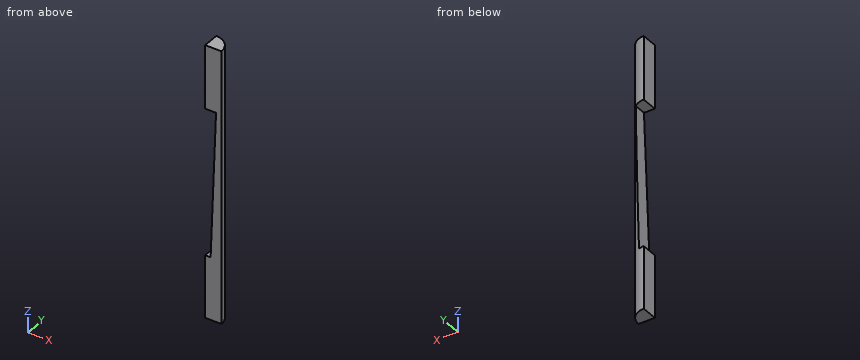
Autodesk Inventor part; units mm, degrees
ref_plane "YZ Plane" through (0, 0, 0) normal (1, 0, 0) x (0, 1, 0)
ref_plane "XZ Plane" through (0, 0, 0) normal (0, 1, 0) x (-1, 0, 0)
ref_plane "XY Plane" through (0, 0, 0) normal (0, 0, 1) x (1, 0, 0)
sketch "Sketch1" plane through (0, 0, 0) normal (0, 0, 1) x (1, 0, 0)
  arc A0 (9.525, 0) -> (0, 9.525) centre (0, 0) ccw
  line L0 (0, 9.525) -> (0, 0)
  line L1 (0, 0) -> (9.525, 0)
  dimension "d0" = 19.05
extrude "Extrusion1" add sketch "Sketch1" along normal mid plane 161.925
sketch "Sketch2" plane through (0, 0, 80.9625) normal (0, -1, 0) x (1, 0, 0)
  line L0 (0, -38.1) -> (6.35, -38.1)
  line L1 (3.175, -123.825) -> (0, -123.825)
  line L2 (0, -123.825) -> (0, -38.1)
  line L3 (9.525, -161.925) -> (0, -161.925)
  line L4 (0, -161.925) -> (0, 0)
  line L5 (3.175, -123.825) -> (6.35, -38.1)
  point P0 (0, -80.9625)
  dimension "d4" = 38.1
  dimension "d8" = 3.175
  dimension "d9" = 6.35
extrude "Extrusion2" cut sketch "Sketch2" against normal through all
sketch "Sketch3" plane through (0, 0, -80.9625) normal (0, -1, 0) x (1, 0, 0)
  line L0 (9.525, 0) -> (0, 0)
  line L1 (0, 0) -> (0, 38.1)
  line L2 (9.525, 0) -> (0, 0)
  line L3 (0, 0) -> (0, 1.4732)
  line L4 (0, 1.4732) -> (9.525, 1.4732)
  line L5 (9.525, 1.4732) -> (9.525, 0)
  line L6 (0, 161.925) -> (9.525, 161.925)
  line L7 (9.525, 161.925) -> (9.525, 0)
  line L8 (0, 161.925) -> (9.525, 161.925)
  line L9 (9.525, 161.925) -> (9.525, 161.0106)
  line L10 (9.525, 161.0106) -> (0, 161.0106)
  line L11 (0, 161.0106) -> (0, 161.925)
  point P0 (0, 80.9625)
  dimension "d10" = 1.4732
  dimension "d11" = 0.9144
extrude "Extrusion3" cut sketch "Sketch3" against normal through all
equation "\"d0\" = cornerRoundType"
equation "\"d1\" = lengthOfPart"
equation "\"d4\" = bottomLength"
equation "\"d8\" = notchDepthLeftSide"
equation "\"d9\" = notchDepthRightSide"
equation "\"d10\" = leftSideLengthRemove"
equation "\"d11\" = rightSideLengthRemove"
equation "\"cornerRoundType\" = 19.05"
equation "\"notchCutout\" = 85.725"
equation "\"bottomLength\" = 38.1"
equation "\"lengthOfPart\" = 2 * bottomLength + notchCutout"
equation "\"notchDepth\" = 6.35"
equation "\"notchDepthLeftSide\" = 3.175"
equation "\"notchDepthRightSide\" = 6.35"
equation "\"leftSideLengthRemove\" = 1.4732"
equation "\"rightSideLengthRemove\" = 0.9144"
properties part number "customMoulding"
Check sheet for the modelled part. Datum: model origin and axes. Units: mm. Coordinates: 2 decimals unless noted, no trailing zeros. Loops run counter-clockwise (first coordinate to the right, second up) from the corner with the lowest first, then second, coordinate; pieces in that order, holes last.
1) Material ranges on probe 1 along Z at (x, y) = (3, 1.25); probe 2 along Y at (x, z) = (1.5, -57.5); probe 3 along X at (y, z) = (1.5, -13), recorded low to high.
2) Sectioned sample at B-B (z = 55). Record the boundary of the cut face in (x, y) (3 decimals), and give its area (3 significant figures).
3) Sectioned sample at C-C (z = 7). Record the boundary of the cut face in (x, y) (3 decimals), and give its area (3 significant figures).
4) Gauge pin test, flat ends, axial feed: pin 1 (1.5 mm diameter, centred on x = 4, z = -17.5, fed in from +Y); pin 2 (5 mm diameter, centred on y = 7.5, z = -35.5, fed in from -X); pin 3 (4 mm diameter, centred on y = 8, z = -38.5, fed in from -X). Record the tip position at first contact, or that the pin passes through.
Check sheet entries:
1. probe 1: z = -79.49 to -42.86, 42.86 to 80.05
1. probe 2: y = 0 to 9.41
1. probe 3: x = 4.28 to 9.41
2. outline: (0, 0) - (9.525, 0) arc R9.525 ccw to (0, 9.525) - close
2. area: 71.3 mm2
3. outline: (5.022, 0) - (9.525, 0) arc R9.525 ccw to (5.022, 8.094) - close
3. area: 25.7 mm2
4. pin 1: stops at y = 8.6
4. pin 2: stops at x = 3.36
4. pin 3: stops at x = 3.26
